Geometry check sheet. Reference: the model listing, model coordinates, mm. A direction names the side the tool comes from. Round coordinates to 2 decimals unless told otherwise and drop trailing zeros. Write each loop counter-clockwise with the first axis right and the second up, starting at its lowest first coordinate (ties: lowest second). Pieces come first, ordered by that corner, then holes. Notation, with made-up numbers: (76.5, -25.75) -> (90.5, -25.75) arc R22 cw to (90.5, -19.75) -> close; hole circle Ø11 at (-28, -5). An arc over 180 degrees is marked (long way). Use a Markdown table: item, result.
```python
from build123d import *

# Parameters (mm, degrees)
SKETCH1_W           = 45
SKETCH1_H           = 20
SKETCH1_R           = 8
SKETCH1_H_2         = 13
SKETCH1_H_3         = 1
BOSS_EXTRUDE1_DEPTH = 3
SKETCH3_W           = 45
SKETCH3_H           = 2.9
SKETCH3_H_2         = 6.2
BOSS_EXTRUDE2_DEPTH = 10
SKETCH3_3_W         = 45
SKETCH3_3_H         = 2.9
BOSS_EXTRUDE3_DEPTH = 22
SKETCH6_R           = 1.525
SKETCH6_W           = 7.6
SKETCH6_H           = 12
CUT_EXTRUDE2_DEPTH  = 16.5
CHAMFER1_SIZE       = 5
FILLET2_R           = 5
FILLET3_SIZE        = 7
FILLET3_SIZE_2      = 6


with BuildPart() as part:
    # Sketch1 → Boss-Extrude1 (new body)
    # profile 1 of 3: a face of its own
    with BuildSketch(Plane(origin=(0, 0, 0), x_dir=(1, 0, 0), z_dir=(0, 1, 0))):
        Rectangle(SKETCH1_W, SKETCH1_H)
        with Locations(Location((13, 0, 0), (0, 0, 270))):
            Circle(SKETCH1_R, mode=Mode.SUBTRACT)
        with Locations(Location((-13, 0, 0), (0, 0, 270))):
            Circle(SKETCH1_R, mode=Mode.SUBTRACT)
    # profile 2 of 3: a face of its own
    with BuildSketch(Plane(origin=(0, 0, 0), x_dir=(1, 0, 0), z_dir=(0, 1, 0))):
        with Locations((0, -16.5)):
            Rectangle(SKETCH1_W, SKETCH1_H_2)
    # profile 3 of 3: a face of its own
    with BuildSketch(Plane(origin=(0, 0, 0), x_dir=(1, 0, 0), z_dir=(0, 1, 0))):
        with Locations((0, -10.5)):
            Rectangle(SKETCH1_W, SKETCH1_H_3)
    extrude(amount=BOSS_EXTRUDE1_DEPTH)

    # Sketch3 → Boss-Extrude2 (add)
    with BuildSketch(Plane(origin=(0, 3, 0), x_dir=(1, 0, 0), z_dir=(0, 1, 0))):
        with Locations((0, -21.55)):
            Rectangle(SKETCH3_W, SKETCH3_H)
        with Locations((0, -17)):
            Rectangle(SKETCH3_W, SKETCH3_H_2)
        with Locations((0, -12.45)):
            Rectangle(SKETCH3_W, SKETCH3_H)
    extrude(amount=BOSS_EXTRUDE2_DEPTH)

    # Sketch3<3> → Boss-Extrude3 (add)
    with BuildSketch(Plane(origin=(0, 3, 0), x_dir=(1, 0, 0), z_dir=(0, 1, 0))):
        with Locations((0, -12.45)):
            Rectangle(SKETCH3_3_W, SKETCH3_3_H)
        with Locations((0, -21.55)):
            Rectangle(SKETCH3_3_W, SKETCH3_3_H)
    extrude(amount=BOSS_EXTRUDE3_DEPTH)

    # Sketch6 → Cut-Extrude2 (cut)
    with BuildSketch(Plane(origin=(0, 0, 11), x_dir=(-1, 0, 0), z_dir=(0, 0, -1))):
        with Locations((-8, 19)):
            Circle(SKETCH6_R)
        with Locations((8, 19)):
            Circle(SKETCH6_R)
        with Locations((-18.7, 19)):
            Rectangle(SKETCH6_W, SKETCH6_H)
        with Locations((18.7, 19)):
            Rectangle(SKETCH6_W, SKETCH6_H)
    extrude(amount=-CUT_EXTRUDE2_DEPTH, mode=Mode.SUBTRACT)

    # Chamfer1
    chamfer1_edges = [part.edges().sort_by_distance(p)[0] for p in [
        (0, 0, 23),
    ]]
    chamfer(chamfer1_edges, length=CHAMFER1_SIZE)

    # Fillet2
    fillet2_edges = [part.edges().sort_by_distance(p)[0] for p in [
        (-22.5, 1.5, -10),
        (22.5, 1.5, -10),
    ]]
    fillet(fillet2_edges, radius=FILLET2_R)

    # Fillet3
    # an asymmetric fillet: 7, 6 mm, written as the material it takes off along each edge
    with BuildSketch(Plane(origin=(14.9, 25, -6.5), x_dir=(-1, 0, 0), z_dir=(0, 0, 1)), Plane(origin=(-14.9, 25, -6.5), x_dir=(0, -1, 0), z_dir=(0, 0, 1))) as fillet3_piece_1:
        with BuildLine():
            Bezier((FILLET3_SIZE, 0), (0, 0), (0, FILLET3_SIZE_2), weights=[1, 0.707106781, 1])
            Line((0, FILLET3_SIZE_2), (0, 0))
            Line((0, 0), (FILLET3_SIZE, 0))
        make_face()
    extrude(amount=37.9, mode=Mode.SUBTRACT)
    with BuildSketch(Plane(origin=(14.9, 25, 2.6), x_dir=(0, -1, 0), z_dir=(0, 0, 1)), Plane(origin=(-14.9, 25, 2.6), x_dir=(1, 0, 0), z_dir=(0, 0, 1))) as fillet3_piece_2:
        with BuildLine():
            Bezier((FILLET3_SIZE_2, 0), (0, 0), (0, -FILLET3_SIZE), weights=[1, 0.707106781, 1])
            Line((0, -FILLET3_SIZE), (0, 0))
            Line((0, 0), (FILLET3_SIZE_2, 0))
        make_face()
    extrude(amount=37.9, mode=Mode.SUBTRACT)


solid = part.part
```
(1) Thickness scan on line 1 (Y direction, x = 8, z = 21) (3 decimals); line 2 (Z direction, x = -13, y = 20.5); line 3 (Y direction, x = 2, z = 17). Record the ranges inside material, lowest first.
A:
| item | result |
|---|---|
| line 1 | y = 3 to 17.475, 20.525 to 24.999 |
| line 2 | z = 11 to 13.9, 20.1 to 23 |
| line 3 | y = 0 to 13 |
(2) Section check D-D on z = 12. State how many separate pieces and enclosed holes the cut face has, plus the area to 3 significant figures.
A:
| item | result |
|---|---|
| separate pieces | 1 |
| enclosed holes | 2 |
| area | 910 mm2 |
(3) Gauge pin test, flat ends, axial feed: pin 1 Ø0.9 at (y, z) = (16.5, 12.5) entering from -X; pin 2 Ø3.5 at (x, y) = (7, 19) entering from -Z; pin 3 Ø1.5 at (x, z) = (3, -2.5) entering from +Y. Record the tip position at first contact, or that the pin passes through.
A:
| item | result |
|---|---|
| pin 1 | stops at x = -14.9 |
| pin 2 | stops at z = 11 |
| pin 3 | stops at y = 3 |
(4) Section check A-A on y = 16.5. Record the cut outline in (x, z).
A:
| item | result |
|---|---|
| outline | (-14.9, 11) -> (14.9, 11) -> (14.9, 13.9) -> (-14.9, 13.9) -> close; (-14.9, 20.1) -> (14.9, 20.1) -> (14.9, 23) -> (-14.9, 23) -> close |
(5) Access from +Z, -Z, +X, -X, +Y, -Y to the whole of each face (thin tool, end or side, straight path). Record for faces 5 (the face through (14.9, 16, 12)), 6 (the face through (21, 1.52, -8.57)), 7 (the face through (-14.9, 15, 12)), 8 (the face through (0, 0, 4)), 9 (the face through (0, 3, 0)).
A:
| item | result |
|---|---|
| face 5 | +Z, -Z, +X, +Y |
| face 6 | -Z, +X, +Y, -Y |
| face 7 | +Z, -Z, -X, +Y |
| face 8 | +Z, -Z, +X, -X, -Y |
| face 9 | -Z, +X, -X, +Y |
(6) Section check C-C on x = -4. Record the cut outline in (y, z), plus the area to 3 significant figures.
A:
| item | result |
|---|---|
| outline | (0, -10) -> (3, -10) -> (3, 11) -> (25, 11) -> (25, 13.9) -> (13, 13.9) -> (13, 20.1) -> (25, 20.1) -> (25, 23) -> (5, 23) -> (0, 18) -> close |
| area | 276 mm2 |
(7) Section check B-B on z = 0. Record the cut outline in (x, y), plus the area to 3 significant figures.
A:
| item | result |
|---|---|
| outline | (-22.5, 0) -> (-21, 0) -> (-21, 3) -> (-22.5, 3) -> close; (-5, 0) -> (5, 0) -> (5, 3) -> (-5, 3) -> close; (21, 0) -> (22.5, 0) -> (22.5, 3) -> (21, 3) -> close |
| area | 39.0 mm2 |
(8) Release check for a two-part mould opening along Z. For faces 1 (the face through (0, 19, 13.9)), 2 (the face through (0, 3, 21)), 3 (the face through (0, 19, 20.1)), 4 (the face through (-14.9, 15, 22)) record: +Z half, -Z half, draft (parallel to the pull), parting line (faces both ways), or undercut.
A:
| item | result |
|---|---|
| face 1 | undercut |
| face 2 | +Z half |
| face 3 | undercut |
| face 4 | draft |
